```python
from build123d import *

# Parameters (mm, degrees)
SKETCH1_W           = 6
SKETCH1_H           = 6
BOSS_EXTRUDE1_DEPTH = 14
HOLE2_D             = 6.5
HOLE1_D             = 6.5
CUT_EXTRUDE2_DEPTH  = 47.465040622
CUT_EXTRUDE1_DEPTH  = 46.814563472
SKETCH8_R           = 3.2
CUT_EXTRUDE3_DEPTH  = 50.746716719
CHAMFER1_SIZE       = 0.5


with BuildPart() as part:
    # Sketch1 → Boss-Extrude1 (new body)
    with BuildSketch(Plane.XY.offset(14)):
        with BuildLine():
            Line((7, 0), (7, 20.267949192))
            Line((7, 20.267949192), (2, 28.92820323))
            Line((2, 28.92820323), (-15.552558883, 39.062177826))
            ThreePointArc((-15.552558883, 39.062177826), (-25.11473671, 36.5), (-22.552558883, 26.937822174))
            Line((-22.552558883, 26.937822174), (-10.464101615, 19.958548116))
            Line((-10.464101615, 19.958548116), (-7, 13.958548116))
            Line((-7, 13.958548116), (-7, 0))
            ThreePointArc((-7, 0), (-6.480740698, -2.645751311), (-5, -4.898979486))
            Line((-5, -4.898979486), (-5, -14))
            Line((-5, -14), (-6, -14))
            Line((-6, -14), (-6, -16))
            Line((-6, -16), (6, -16))
            Line((6, -16), (6, -14))
            Line((6, -14), (5, -14))
            Line((5, -14), (5, -4.898979486))
            ThreePointArc((5, -4.898979486), (6.480740698, -2.645751311), (7, 0))
        make_face()
        with Locations((0, -11)):
            Rectangle(SKETCH1_W, SKETCH1_H, mode=Mode.SUBTRACT)
    extrude(amount=-BOSS_EXTRUDE1_DEPTH)

    # Hole2 (through all)
    with Locations(Plane(origin=(0, 0, 0), x_dir=(-1, 0, 0), z_dir=(0, 0, -1))):
        with Locations((19.0525, 32.999898011)):
            Hole(HOLE2_D / 2)

    # Hole1 (through all)
    with Locations(Plane(origin=(0, 0, 0), x_dir=(-1, 0, 0), z_dir=(0, 0, -1))):
        with Locations((0, 0)):
            Hole(HOLE1_D / 2)

    # Sketch3 → Cut-Extrude2 (cut, through all)
    with BuildSketch(Plane.ZY.offset(7)):
        with BuildLine():
            Line((9.298097039, 4.701902961), (11.596194078, 7))
            Line((11.596194078, 7), (9.298097039, 9.298097039))
            ThreePointArc((9.298097039, 9.298097039), (3.75, 7), (9.298097039, 4.701902961))
        make_face()
    extrude(amount=-CUT_EXTRUDE2_DEPTH, mode=Mode.SUBTRACT)

    # Sketch2 → Cut-Extrude1 (cut, through all)
    with BuildSketch(Plane(origin=(6.026279442, 10.437822174, 0), x_dir=(0.8660254037844398, -0.49999999999999806, 0), z_dir=(-0.499999999999998, -0.8660254037844397, 0))):
        with BuildLine():
            Line((-25.999898011, 11.596194078), (-28.29799505, 9.298097039))
            ThreePointArc((-28.29799505, 9.298097039), (-25.999898011, 3.75), (-23.701800972, 9.298097039))
            Line((-23.701800972, 9.298097039), (-25.999898011, 11.596194078))
        make_face()
    extrude(amount=-CUT_EXTRUDE1_DEPTH, mode=Mode.SUBTRACT)

    # Sketch8 → Cut-Extrude3 (cut, through all)
    with BuildSketch(Plane.XY.offset(14)):
        with Locations((-2.116025404, 20.778312164)):
            Circle(SKETCH8_R)
    extrude(amount=-CUT_EXTRUDE3_DEPTH, mode=Mode.SUBTRACT)

    # Chamfer1
    chamfer1_edges = [part.edges().sort_by_distance(p)[0] for p in [
        (4.5, 24.598076211, 0),
        (-6.776279442, 33.995190528, 0),
        (-25.11473671, 36.5, 0),
        (-16.508330249, 23.448185145, 0),
        (-8.732050808, 16.958548116, 0),
        (-7, 6.979274058, 0),
        (-6.480740698, -2.645751311, 0),
        (-5, -9.449489743, 0),
        (-5.5, -14, 0),
        (-6, -15, 0),
        (6.480740698, -2.645751311, 0),
        (0, -16, 0),
        (-3, -11, 0),
        (0, -8, 0),
        (3, -11, 0),
        (0, -14, 0),
        (6, -15, 0),
        (5.5, -14, 0),
        (5, -9.449489743, 0),
        (-22.3025, 32.999898011, 0),
        (-3.25, 0, 0),
        (7, 10.133974596, 0),
        (-5.316025404, 20.778312164, 0),
    ]]
    chamfer(chamfer1_edges, length=CHAMFER1_SIZE)


solid = part.part
```
Input: part model. Units: mm. Frame: model coordinates. A direction names the side the tool comes from. Give positions to 0.01 mm unless a question says otherwise; leave off trailing zeros. Order: outer loops, then holes, each group sorted by start corner. A loop starts at its lowest first (then second) coordinate and runs counter-clockwise, first axis right, second up. Notation, with made-up numbers: (61.5, 14.5) - (94.5, 14.5) arc R11 cw to (94.5, 26.5) - close; hole circle Ø10 at (67, 63.5). An arc over 180 degrees is marked (long way). One line per item, written item: value.
1. Draft query along Y for faces 5 (the face through (0, -16, 7)), 6 (the face through (-6, 18, 0)), 7 (the face through (-12.03, 28.83, 10.43)). Return one class per face: released by +Y, released by -Y, zero draft, split by the parting line, or undercut.
Determined:
face 5: released by -Y
face 6: zero draft
face 7: undercut
2. Reachability of faces 1 (the face through (6.466, -2.681, 7.344)), 2 (the face through (-14.02, 29.982, 10.463)), 3 (the face through (-6, -15, 7)), 4 (the face through (-0.098, 8.133, 10.463)) from +Z, -Z, +X, -X, +Y, -Y: full face, straight path, thin tool, end or side. Return the list, or none.
Determined:
face 1: +Z, -Z, +X
face 2: none
face 3: +Z, -Z, -X, -Y
face 4: +X, -X
3. Cut plane B-B, the plane y = 13. Output: boundary loops of the cut face in (x, z), and give its area (3 significant figures).
Determined:
outline: (-7, 0.5) - (-6.5, 0) - (6.5, 0) - (7, 0.5) - (7, 14) - (-7, 14) - close
area: 196 mm2
4. Line query: probe 1 along Y at (x, z) = (-2.5, 2.25); probe 2 along X at (y, z) = (31.5, 11.25); probe 3 along X at (y, z) = (-9, 2.75). Output: solid intervals per line, ascending.
Determined:
probe 1: -16 to -14, -8 to -2.08, 2.08 to 17.6, 23.96 to 31.53
probe 2: -25.89 to -21.94, -16.17 to -12.24, -11.44 to -2.45
probe 3: -5 to -3, 3 to 5
5. Cut plane A-A, the plane z = 11. Give the number of separate pieces and of enclosed holes in the cut face, and give its area (3 significant figures).
Determined:
separate pieces: 3
enclosed holes: 4
area: 695 mm2
6. Pin query (flat end, axial travel): pin 1 Ø6.5 at (y, z) = (-11.5, 7) entering from +X; pin 2 Ø2.5 at (y, z) = (-7.5, 4.5) entering from +X; pin 3 Ø7.5 at (y, z) = (-9.5, 5) entering from -X; pin 4 Ø5 at (x, y) = (0, 0) entering from -Z. Return the tip coordinate at first contact, or that it passes through.
Determined:
pin 1: x = 6
pin 2: x = 5
pin 3: x = -5
pin 4: through
